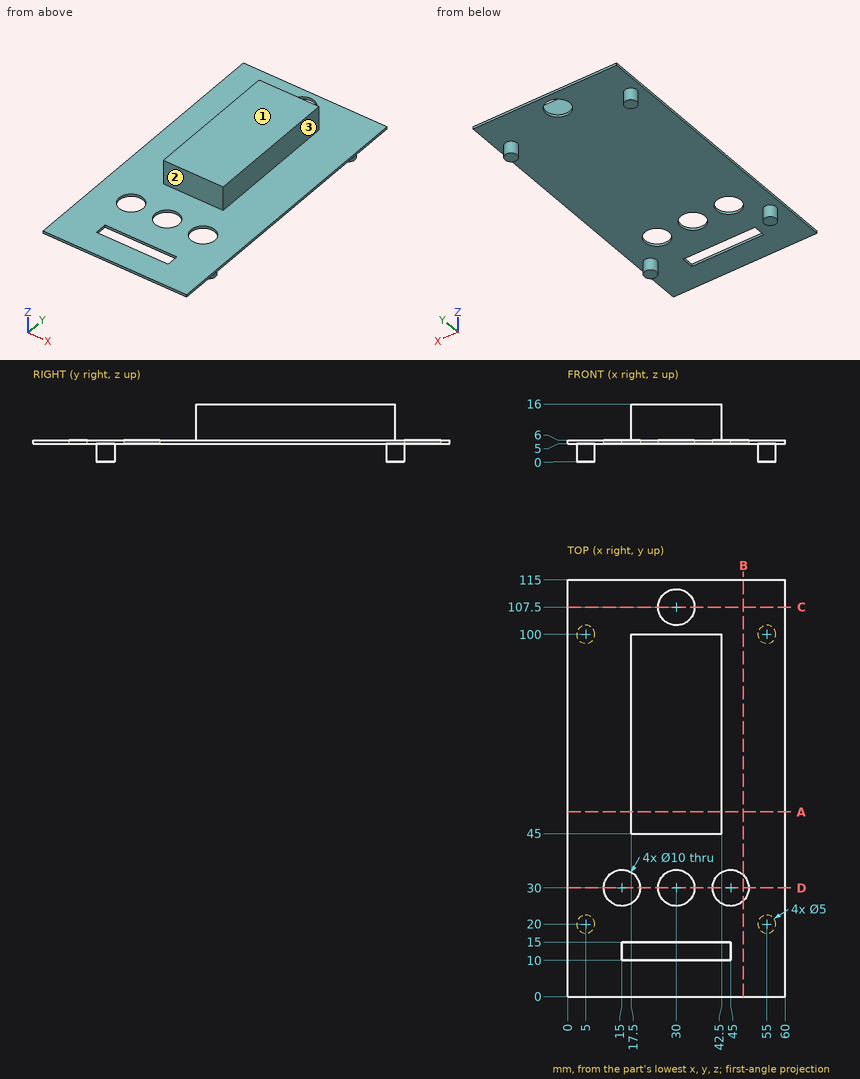
For this review, use the dimensioned drawing (mm, ordinates from the lowest corner) and the shaded views. A direction names the side the tool comes from. Give positions to 0.01 mm unless a question says otherwise; leave off trailing zeros. Write each loop counter-clockwise with the first axis right and the second up, starting at its lowest first coordinate (ties: lowest second). Pieces come first, ordered by that corner, then holes. Notation, with made-up numbers: M -15,39.25 L -3,39.25 A15 cw -3,68.25 Z; hole C -40,84.25 d4. An arc over 180 degrees is marked long. Write item = value, one per line. Start each with the question number.
Q1. Clearance check with flat-ended pins moving along their axes: pin 1 (5 mm diameter, centred on x = 36, z = 13, fed in from -Y); pin 2 (3 mm diameter, centred on y = 81.5, z = 13, fed in from -X); pin 3 (1 mm diameter, centred on x = 16, y = 90.5, fed in from -Z); pin 4 (4 mm diameter, centred on x = 46.5, z = 7, fed in from +Y). State where each tip first meets the part, or that it passes through.
Q2. Machinability: for the marked faces 1, 2 and 3, which of the approach directions +Z, -Z, +X, -X, +Y, -Y give a long, thin tool a straight path to every point of the face, cutting with its end or side? Answer none if there is none.
Q3. We need section C-C (y = 107.5). State the section outline as (x, z) points, plus the area to 3 significant figures.
Q4. We need section D-D (y = 30). State the section outline as (x, z) points, plus the area to 3 significant figures.
Q5. We need section B-B (x = 48.5). State the section outline as (y, z) points, plus the area to 3 significant figures.
Q6. For line 1 (Y direction, x = 30, z = 5.65); line 2 (Z direction, x = 38, y = 35); line 3 (X direction, y = 93, z = 13.5), list the stretches that pass through material, from the lowest coordinate up.
Q7. We need section A-A (y = 51). State the section outline as (x, z) points, plus the area to 3 significant figures.
Result set:
q1.pin_1 = 45
q1.pin_2 = 17.5
q1.pin_3 = 5
q1.pin_4 = 115
q2.face_1 = +Z, +X, -X, +Y, -Y
q2.face_2 = +Z, +X, -X, -Y
q2.face_3 = +Z, +X, +Y, -Y
q3.outline = M 0,5 L 25,5 L 25,6 L 0,6 Z; M 35,5 L 60,5 L 60,6 L 35,6 Z
q3.area = 50.0 mm2
q4.outline = M 0,5 L 10,5 L 10,6 L 0,6 Z; M 20,5 L 25,5 L 25,6 L 20,6 Z; M 35,5 L 40,5 L 40,6 L 35,6 Z; M 50,5 L 60,5 L 60,6 L 50,6 Z
q4.area = 30.0 mm2
q5.outline = M 0,5 L 26.43,5 L 26.43,6 L 0,6 Z; M 33.57,5 L 115,5 L 115,6 L 33.57,6 Z
q5.area = 108 mm2
q6.line_1 = 0 to 10, 15 to 25, 35 to 102.5, 112.5 to 115
q6.line_2 = 5 to 6
q6.line_3 = 17.5 to 42.5
q7.outline = M 0,5 L 60,5 L 60,6 L 42.5,6 L 42.5,16 L 17.5,16 L 17.5,6 L 0,6 Z
q7.area = 310 mm2
